```python
from build123d import *

# Parameters (mm, degrees)
SALIENTE_EXTRUIR1_DEPTH = 16
CORTAR_EXTRUIR1_REACH   = 18
CROQUIS2_W              = 6.2
CROQUIS2_H              = 6.2
CORTAR_EXTRUIR2_REACH   = 24.5
CROQUIS3_R              = 1.6
CORTAR_EXTRUIR3_DEPTH   = 3
CORTAR_EXTRUIR4_REACH   = 46.5
CROQUIS5_R              = 1.6
CORTAR_EXTRUIR5_DEPTH   = 3


with BuildPart() as part:
    # Croquis1 → Saliente-Extruir1 (new body)
    with BuildSketch(Plane.XY):
        Polygon((0, 0), (0, 1.7), (2, 1.7), (2, 21.7), (5, 21.7), (5, 39.7), (2, 39.7), (2, 50.7), (9, 50.7), (9, 10), (24.5, 10), (24.5, 0), align=None)
    extrude(amount=SALIENTE_EXTRUIR1_DEPTH)

    # Croquis2 → Cortar-Extruir1 (cut, up to next)
    with BuildSketch(Plane.XY.offset(16), mode=Mode.PRIVATE) as cortar_extruir1_sk1:
        with Locations((21.4, 3.1)):
            Rectangle(CROQUIS2_W, CROQUIS2_H)
    cortar_extruir1_tool1 = extrude(cortar_extruir1_sk1.sketch, amount=-CORTAR_EXTRUIR1_REACH, mode=Mode.PRIVATE) & part.part
    add(cortar_extruir1_tool1.solids().sort_by_distance((21.4, 3.1, 16))[0], mode=Mode.SUBTRACT)

    # Croquis3 → Cortar-Extruir2 (cut, up to next)
    with BuildSketch(Plane.ZY.offset(-2), mode=Mode.PRIVATE) as cortar_extruir2_sk1:
        with Locations((3.5, 45.1)):
            Circle(CROQUIS3_R)
    cortar_extruir2_tool1 = extrude(cortar_extruir2_sk1.sketch, amount=-CORTAR_EXTRUIR2_REACH, mode=Mode.PRIVATE) & part.part
    add(cortar_extruir2_tool1.solids().sort_by_distance((2, 45.1, 3.5))[0], mode=Mode.SUBTRACT)

    # Croquis4 → Cortar-Extruir3 (cut)
    with BuildSketch(Plane(origin=(9, 0, 0), x_dir=(0, 0, -1), z_dir=(1, 0, 0))):
        Polygon((-0.65, 46.745448267), (-3.5, 48.390896534), (-6.35, 46.745448267), (-6.35, 43.454551733), (-3.5, 41.809103466), (-0.65, 43.454551733), align=None)
    extrude(amount=-CORTAR_EXTRUIR3_DEPTH, mode=Mode.SUBTRACT)

    # Croquis5 → Cortar-Extruir4 (cut, up to next)
    with BuildSketch(Plane.XZ.offset(-6.2), mode=Mode.PRIVATE) as cortar_extruir4_sk1:
        with Locations((21.4, 11.62)):
            Circle(CROQUIS5_R)
    cortar_extruir4_tool1 = extrude(cortar_extruir4_sk1.sketch, amount=-CORTAR_EXTRUIR4_REACH, mode=Mode.PRIVATE) & part.part
    add(cortar_extruir4_tool1.solids().sort_by_distance((21.4, 6.2, 11.62))[0], mode=Mode.SUBTRACT)

    # Croquis6 → Cortar-Extruir5 (cut)
    with BuildSketch(Plane(origin=(0, 10, 0), x_dir=(1, 0, 0), z_dir=(0, 1, 0))):
        Polygon((19.754551733, -14.47), (23.045448267, -14.47), (24.690896534, -11.62), (23.045448267, -8.77), (19.754551733, -8.77), (18.109103466, -11.62), align=None)
    extrude(amount=-CORTAR_EXTRUIR5_DEPTH, mode=Mode.SUBTRACT)


solid = part.part
```
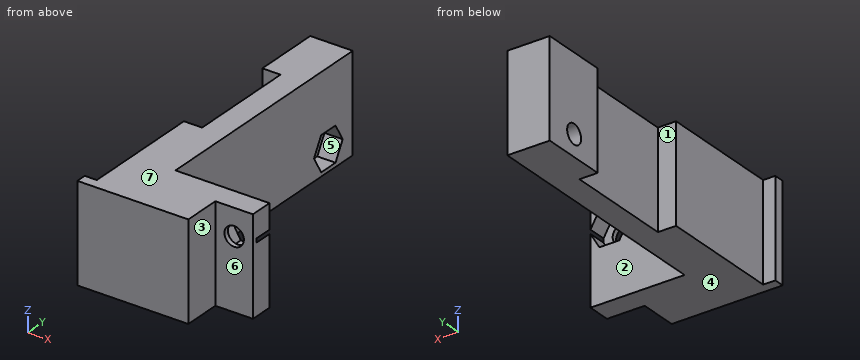
Verification items for the finished model (mm, model axes). Face numbers are marked on the shaded views. A direction names the side the tool comes from. Round coordinates to 2 decimals unless told otherwise and drop trailing zeros. Order: outer loops, then holes, each group sorted by start corner. A loop starts at its lowest first (then second) coordinate and runs counter-clockwise, first axis right, second up. Notation, with made-up numbers: (84, 45) - (95, 45) arc R36 cw to (95, 79) - close; hole circle Ø1 at (29, 39.25). An arc over 180 degrees is marked (long way). Use CSV: the item, a comma, the result in double quotes. Start each with the question number.
1) Mould release check, pull along Z, two halves, no side actions. Record for the marked faces 4, 5, 6 and 7: +Z half, -Z half, draft (parallel to the pull), parting line (faces both ways), or undercut.
2) Thickness scan on L1, parallel to Y at x = 3.5, z = 3.5; L2, parallel to Y at x = 2.5, z = 6.5; L3, parallel to X at y = 21.5, z = 7.75. Record the ranges inside material, lowest first.
3) Go/stop test with flat-tipped pins: P1, Ø8, axis at x = 15, z = 7.5, coming from the +Y side; P2, Ø8, axis at y = 14, z = 9.5, coming from the -X side; P3, Ø3, axis at x = 21.5, z = 8.5, coming from the -Y side. Record where each tip stops, or that it passes through.
4) Section check A-A, the plane y = 45.1. Record the cut outline in (x, z), plus the area to 3 significant figures.
5) Access from +Z, -Z, +X, -X, +Y, -Y to the whole of each face (thin tool, end or side, straight path). Record for the marked faces 1, 2 and 3.
6) Section check D-D, the plane y = 16.5. Record the cut outline in (x, z), plus the area to 3 significant figures.
7) Section check B-B, the plane x = 21.4. Record the cut outline in (y, z).
8) Section check C-C, the plane z = 10.75. Record the cut outline in (x, y).
Answers:
1,face 4,"-Z half"
1,face 5,"undercut"
1,face 6,"draft"
1,face 7,"+Z half"
2,L1,"y = 0 to 21.7, 39.7 to 43.5, 46.7 to 50.7"
2,L2,"y = 0 to 21.7, 39.7 to 50.7"
2,L3,"x = 2 to 9"
3,P1,"stops at y = 10"
3,P2,"stops at x = 2"
3,P3,"stops at y = 6.2"
4,outline,"(2, 0) - (9, 0) - (9, 0.65) - (6, 0.65) - (6, 1.9) - (2, 1.9) - close; (2, 5.1) - (6, 5.1) - (6, 6.35) - (9, 6.35) - (9, 16) - (2, 16) - close"
4,area,"82.1 mm²"
5,face 1,"+Z, -Z, -X"
5,face 2,"+Z, -Z, +X, +Y"
5,face 3,"+Z, -Z, +X, -Y"
6,outline,"(2, 0) - (9, 0) - (9, 16) - (2, 16) - close"
6,area,"112 mm²"
7,outline,"(6.2, 0) - (10, 0) - (10, 8.77) - (7, 8.77) - (7, 10.02) - (6.2, 10.02) - close; (6.2, 13.22) - (7, 13.22) - (7, 14.47) - (10, 14.47) - (10, 16) - (6.2, 16) - close"
8,outline,"(0, 0) - (18.3, 0) - (18.3, 6.2) - (20.06, 6.2) - (20.06, 7) - (18.61, 7) - (18.61, 10) - (9, 10) - (9, 50.7) - (2, 50.7) - (2, 39.7) - (5, 39.7) - (5, 21.7) - (2, 21.7) - (2, 1.7) - (0, 1.7) - close; (22.74, 6.2) - (24.5, 6.2) - (24.5, 10) - (24.19, 10) - (24.19, 7) - (22.74, 7) - close"
